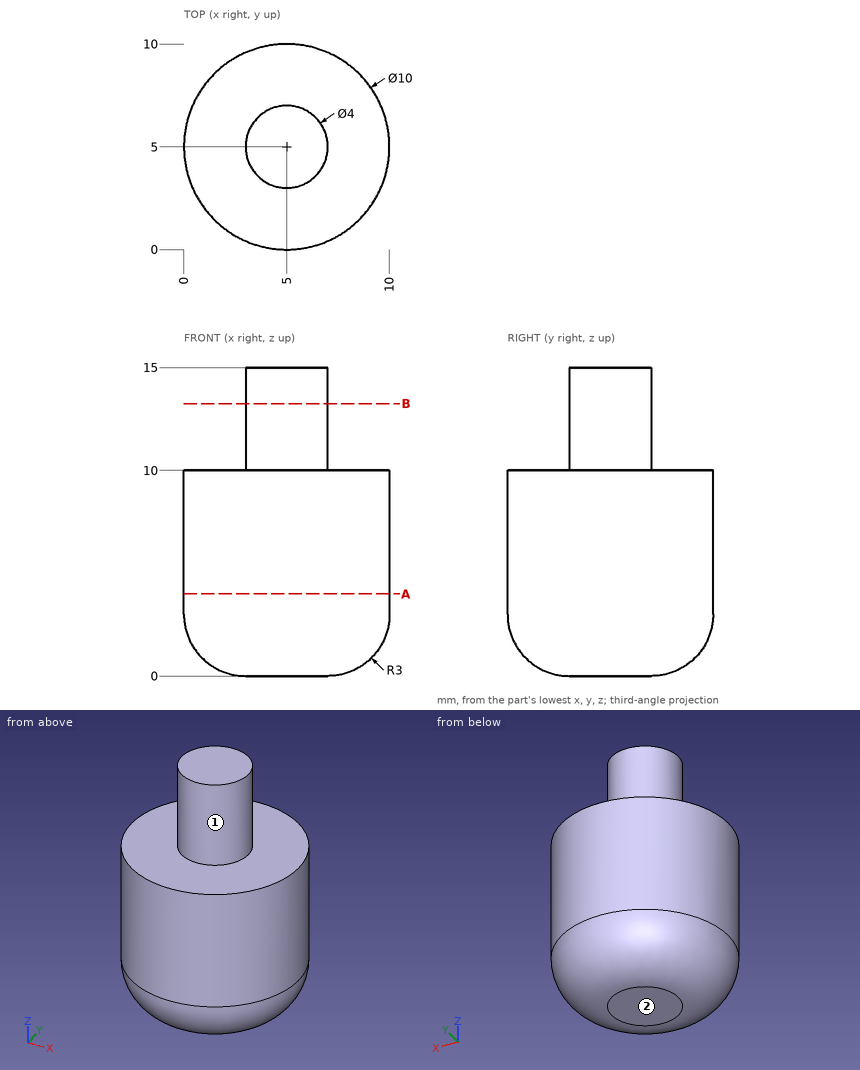
Input: dimensioned drawing with shaded views. Units: mm. Origin: part minimum x, y, z. A direction names the side the tool comes from. Give positions to 0.01 mm unless a question says otherwise; leave off trailing zeros. Order: outer loops, then holes, each group sorted by start corner. A loop starts at its lowest first (then second) coordinate and runs counter-clockwise, first axis right, second up.
(1) Access query for the marked faces 1 and 2. Directions: +Z, -Z, +X, -X, +Y, -Y. A direction counts if a zero-diameter tool reaches every point of the face in a straight line with its end or side. Return the directions, or none.
(2) Contact query for flat-ended pins moving along their axis: P1, Ø2, axis at y = 3, z = 13.5, coming from the -X side; P2, Ø2, axis at x = 2.5, z = 12.5, coming from the -Y side; P3, Ø1.5, axis at x = 1.5, y = 3, coming from the -Z side. Output: stop coordinate, or through.
(3) Section query A-A (z = 4). Return the cut outline in (x, y), plus the area to 3 significant figures.
(4) Material intervals for line 1 along Y through (x, z) = (5, 14.25); line 2 along Y through (x, z) = (5.75, 1.25); line 3 along X through (y, z) = (9.5, 3), sorted ascending.
(5) Section query B-B (z = 13.25). Return the cut outline in (x, y), plus the area to 3 significant figures.
Outcome:
1. face 1: +Z
1. face 2: -Z, +X, -X, +Y, -Y
2. P1: stops at x = 3.27
2. P2: stops at y = 3.68
2. P3: stops at z = 0.29
3. outline: circle Ø10 at (5, 5)
3. area: 78.5 mm2
4. line 1: y = 3 to 7
4. line 2: y = 0.63 to 9.37
4. line 3: x = 2.82 to 7.18
5. outline: circle Ø4 at (5, 5)
5. area: 12.6 mm2
